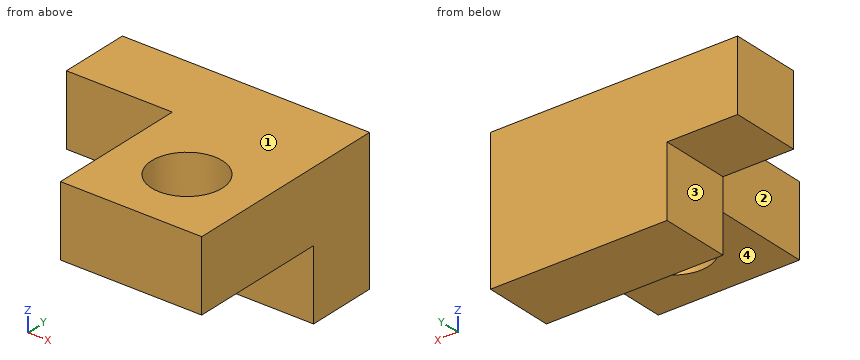
from build123d import *

# Parameters (mm, degrees)
F0_W     = 20
F0_H     = 10
F1_DEPTH = 20
F2_DEPTH = 10
F4_D     = 10


with BuildPart() as f1:
    # F0 (on Front) → F1 (new body)
    with BuildSketch(Plane.XZ):
        with Locations((15, 15)):
            Rectangle(F0_W, F0_H)
    extrude(amount=F1_DEPTH)

    # F0 (on Front) → F2 (join)
    with BuildSketch(Plane.XZ):
        Polygon((0, 10), (0, 0), (25, 0), (25, 10), (5, 10), (5, 20), (-10, 20), (-10, 10), align=None)
        with Locations((15, 15)):
            Rectangle(F0_W, F0_H)
    extrude(amount=-F2_DEPTH)

    # F4 (through all)
    with Locations(Plane(origin=(0, 0, 10), x_dir=(1, 0, 0), z_dir=(0, 0, -1))):
        with Locations((15, 10)):
            Hole(F4_D / 2)


solid = f1.part
Source: CAD feature listing. Evaluate the final solid. Frame: model axes, mm. Face numbers are marked on the shaded views. A direction names the side the tool comes from. Give positions to 0.01 mm unless a question says otherwise; leave off trailing zeros. Write each loop counter-clockwise with the first axis right and the second up, starting at its lowest first coordinate (ties: lowest second). Pieces come first, ordered by that corner, then holes. Notation, with made-up numbers: (-23, 73.5) -> (30, 73.5) arc R17 cw to (30, 93.5) -> close; hole circle Ø4 at (18, 25). An arc over 180 degrees is marked (long way). Write item = value, one per line.
Q1. Reachability of the marked faces 1, 2, 3 and 4 from +Z, -Z, +X, -X, +Y, -Y: full face, straight path, thin tool, end or side. Return the list, or none.
Here are the results:
face_1 = +Z, +X, -X, +Y, -Y
face_2 = +Z, -Z, -X, -Y
face_3 = -Z, -X, +Y, -Y
face_4 = -Z, +X, -X, -Y
Q2. First-contact query: pin 1 (13 mm diameter, centred on x = 15, y = -10, fed in from +Z); pin 2 (6 mm diameter, centred on x = -1, z = 10, fed in from -Y); pin 3 (1.5 mm diameter, centred on y = 6, z = 3.5, fed in from -X); pin 4 (11 mm diameter, centred on y = -12, z = 16.5, fed in from -X). Flat tips, straight axial feed; report the tip coordinate or a pass-through.
Here are the results:
pin_1 = 20
pin_2 = 0
pin_3 = 0
pin_4 = 5
Q3. Cut plane C-C on x = 11.5. Return loops of the section in (y, z).
Here are the results:
outline = (-20, 10) -> (-13.57, 10) -> (-13.57, 20) -> (-20, 20) -> close; (-6.43, 10) -> (0, 10) -> (0, 0) -> (10, 0) -> (10, 20) -> (-6.43, 20) -> close
Q4. Cut plane D-D on y = 7. Return loops of the section in (x, z), then the cut area to 3 significant figures.
Here are the results:
outline = (-10, 10) -> (0, 10) -> (0, 0) -> (25, 0) -> (25, 20) -> (-10, 20) -> close
area = 600 mm²
Q5. Cut plane B-B on z = 13.75. Return loops of the section in (x, y), then the cut area to 3 significant figures.
Here are the results:
outline = (-10, 0) -> (5, 0) -> (5, -20) -> (25, -20) -> (25, 10) -> (-10, 10) -> close; hole circle Ø10 at (15, -10)
area = 671 mm²
Q6. Line query: line 1 (Y direction, x = 15, z = 13.5); line 2 (Z direction, x = 13, y = -17.5); line 3 (X direction, y = 0.25, z = 3.5). Output: solid intervals per line, ascending. Write a range as from..to.
Here are the results:
line_1 = -20..-15, -5..10
line_2 = 10..20
line_3 = 0..25
Q7. Cut plane A-A on y = -10. Return loops of the section in (x, z).
Here are the results:
outline = (5, 10) -> (10, 10) -> (10, 20) -> (5, 20) -> close; (20, 10) -> (25, 10) -> (25, 20) -> (20, 20) -> close
